```python
from build123d import *

# Parameters (mm, degrees)
SALIENTE_EXTRUIR1_DEPTH = 3.302
CROQUIS2_R              = 4.445
CORTAR_EXTRUIR1_DEPTH   = 3.302
MATRIZC1_COUNT          = 4
MATRIZC1_ANGLE          = 180
REDONDEO1_R             = 1.27


with BuildPart() as part:
    # Croquis1 → Saliente-Extruir1 (new body)
    with BuildSketch(Plane.XY):
        with BuildLine():
            Line((-38.1, 0), (-53.34, 0))
            ThreePointArc((-53.34, 0), (0, 53.34), (53.34, 0))
            Line((53.34, 0), (38.1, 0))
            ThreePointArc((38.1, 0), (0, 38.1), (-38.1, 0))
        make_face()
    extrude(amount=SALIENTE_EXTRUIR1_DEPTH)

    # Croquis2 → Cortar-Extruir1 (cut)
    with BuildSketch(Plane.XY.offset(3.302)):
        with Locations((-45.72, 0)):
            Circle(CROQUIS2_R)
    cortar_extruir1 = extrude(amount=-CORTAR_EXTRUIR1_DEPTH, mode=Mode.SUBTRACT)

    # MatrizC1: Cortar-Extruir1 ×4 about axis
    matrizc1_axis = Axis((0, 0, 0), (0, 0, -1))
    for i in range(1, MATRIZC1_COUNT):
        add(cortar_extruir1.rotate(matrizc1_axis, i * MATRIZC1_ANGLE / (MATRIZC1_COUNT - 1)), mode=Mode.SUBTRACT)

    # Redondeo1
    redondeo1_edges = [part.edges().sort_by_distance(p)[0] for p in [
        (-50.165, 0, 1.651),
        (-41.275, 0, 1.651),
        (-38.1, 0, 1.651),
        (-53.34, 0, 1.651),
        (53.34, 0, 1.651),
        (38.1, 0, 1.651),
    ]]
    fillet(redondeo1_edges, radius=REDONDEO1_R)


solid = part.part
```
Here's how the part is built. I have some questions about the finished solid (model axes, mm). Round coordinates to 2 decimals unless told otherwise and drop trailing zeros. Loops run counter-clockwise (first coordinate to the right, second up) from the corner with the lowest first, then second, coordinate; pieces in that order, holes last. Notation, with made-up numbers: (31.5, 59) -> (65.5, 59) arc R15 cw to (65.5, 65) -> close; hole circle Ø11 at (-1, -13). An arc over 180 degrees is marked (long way). Answer as CSV lines item,"result".
1. If we section it at D-D on z = 1.3: Please give me the cut outline in (x, y) (1 decimal), plus the area to 3 significant figures.
Final values:
outline,"(-53.3, 1.3) arc R1.3 ccw to (-52.1, 0) -> (-51.3, 0) arc R1.3 ccw to (-50.1, 1) arc R4.4 cw to (-41.4, 1) arc R1.3 ccw to (-40.1, 0) -> (-39.3, 0) arc R1.3 ccw to (-38.1, 1.2) arc R38.1 cw to (38.1, 1.2) arc R1.3 ccw to (39.3, 0) -> (41.3, 0) arc R4.4 cw to (50.2, 0) -> (52.1, 0) arc R1.3 ccw to (53.3, 1.3) arc R53.3 ccw to start; hole circle Ø8.9 at (-22.9, 39.6); hole circle Ø8.9 at (22.9, 39.6)"
area,"2,000 mm^2"
2. If we section it at A-A on y = 43: Please give me the cut outline in (x, z).
Final values:
outline,"(-31.56, 0) -> (-25.72, 0) -> (-25.72, 3.3) -> (-31.56, 3.3) -> close; (-20, 0) -> (20, 0) -> (20, 3.3) -> (-20, 3.3) -> close; (25.72, 0) -> (31.56, 0) -> (31.56, 3.3) -> (25.72, 3.3) -> close"
3. If I drill on L1, parallel to Y at x = 22.86, z = 1.2; L2, parallel to X at y = 16.5, z = 3.15; L3, parallel to X at y = 32.5, z = 1.5, over which ranges is the centre line in solid material (lowest first)?
Final values:
L1,"y = 30.48 to 35.15, 44.04 to 48.19"
L2,"x = -50.72 to -34.34, 34.34 to 50.72"
L3,"x = -42.3 to -19.88, 19.88 to 42.3"
4. If we section it at B-B on x = -22.86: Please give me the cut outline in (y, z), plus the area to 3 significant figures.
Final values:
outline,"(30.48, 0) -> (35.15, 0) -> (35.15, 3.3) -> (30.48, 3.3) -> close; (44.04, 0) -> (48.19, 0) -> (48.19, 3.3) -> (44.04, 3.3) -> close"
area,"29.1 mm^2"
5. Thinking about a two-plate mould opening in X: for faces 1 (the face through (0, 39, 3.302)), 2 (the face through (-1.155, 53.328, 1.628)), 3 (the face through (45.818, 4.444, 1.674)), which applies, released by +X, released by -X, zero draft, split by the parting line, or undercut?
Final values:
face 1,"zero draft"
face 2,"split by the parting line"
face 3,"undercut"
6. For pin 1 (5.5 mm diameter, centred on x = 22.86, y = 39.59, fed in from -Z), with a flat end and sliding along its axis, tell me the tip position at first contact or that it passes through.
Final values:
pin 1,"passes through"
7. If we section it at C-C on y = 24.5: Please give me the cut outline in (x, z), plus the area to 3 significant figures.
Final values:
outline,"(-47.38, 0) -> (-29.18, 0) -> (-29.18, 3.3) -> (-47.38, 3.3) -> close; (29.18, 0) -> (47.38, 0) -> (47.38, 3.3) -> (29.18, 3.3) -> close"
area,"120 mm^2"
